from build123d import *

# Parameters (mm, degrees)
SKETCH_1_W      = 260
SKETCH_1_H      = 150
SKETCH_1_R      = 21.5
EXTRUDE_1_DEPTH = 5
FILLET_1_R      = 10


with BuildPart() as part:
    # Эскиз1 → Бобышка-Вытянуть1 (new, symmetric)
    with BuildSketch(Plane.XY):
        Rectangle(SKETCH_1_W, SKETCH_1_H)
        Circle(SKETCH_1_R, mode=Mode.SUBTRACT)
    extrude(amount=EXTRUDE_1_DEPTH, both=True)

    # Скругление1
    fillet_1_edges = [part.edges().sort_by_distance(p)[0] for p in [
        (130, -75, 0),
        (-130, -75, 0),
        (-130, 75, 0),
        (130, 75, 0),
    ]]
    fillet(fillet_1_edges, radius=FILLET_1_R)


solid = part.part
Can you work these out from the model? Positions are in its coordinate system, mm. Round coordinates to 2 decimals unless told otherwise and drop trailing zeros. Write each loop counter-clockwise with the first axis right and the second up, starting at its lowest first coordinate (ties: lowest second). Pieces come first, ordered by that corner, then holes. Notation, with made-up numbers: (84, 66.5) -> (132, 66.5) arc R24 cw to (132, 103.5) -> close; hole circle Ø2 at (87.25, -1). An arc over 180 degrees is marked (long way). One line per question, with ' | ' between items. Start each with the question number.
1) If we mould it in two halves opening along Y, with no side actions, what happens to faces 1 (the flat face through (130, -1, 0)), 2 (the cylindrical face through (-2.799, 21.317, -0.07)), 3 (the flat face through (-2, -75, 0)), 4 (the flat face through (-2, 75, 0))? For each: released by +Y, released by -Y, zero draft, split by the parting line, or undercut.
2) Suppose I cut it at A-A on y = 0. Write out the boundary of the cut face in (x, z), then the cut area to 3 significant figures.
3) Suppose I cut it at B-B on x = 0. Write out the boundary of the cut face in (y, z).
4) I need wall thicknesses on line 1 (Y direction, x = 0, z = 1); line 2 (X direction, y = -2.5, z = 0.75); line 3 (Y direction, x = -6, z = 4.25). Which ranges of each line are inside material? Lowest first, please. Write a range as [from, to].
5) Suppose I cut it at C-C on z = 0.75. Write out the boundary of the cut face in (x, y), then the cut area to 3 significant figures.
Return value:
1) face 1: zero draft | face 2: undercut | face 3: released by -Y | face 4: released by +Y
2) outline: (-130, -5) -> (-21.5, -5) -> (-21.5, 5) -> (-130, 5) -> close; (21.5, -5) -> (130, -5) -> (130, 5) -> (21.5, 5) -> close | area: 2,170 mm2
3) outline: (-75, -5) -> (-21.5, -5) -> (-21.5, 5) -> (-75, 5) -> close; (21.5, -5) -> (75, -5) -> (75, 5) -> (21.5, 5) -> close
4) line 1: y = [-75, -21.5], [21.5, 75] | line 2: x = [-130, -21.35], [21.35, 130] | line 3: y = [-75, -20.65], [20.65, 75]
5) outline: (-130, -65) arc R10 ccw to (-120, -75) -> (120, -75) arc R10 ccw to (130, -65) -> (130, 65) arc R10 ccw to (120, 75) -> (-120, 75) arc R10 ccw to (-130, 65) -> close; hole circle Ø43 at (0, 0) | area: 37,500 mm2
